Can you work these out from the model? Positions are in its coordinate system, mm. A direction names the side the tool comes from. Give positions to 0.01 mm unless a question says otherwise; leave off trailing zeros. Loops run counter-clockwise (first coordinate to the right, second up) from the corner with the lowest first, then second, coordinate; pieces in that order, holes last. Notation, with made-up numbers: (53.25, -9.75) -> (57.25, -9.75) arc R13 ccw to (57.25, 7.25) -> close; hole circle Ø9 at (-12, 11). An arc over 180 degrees is marked (long way). One line per question, with ' | ' between items.
from build123d import *

# Parameters (mm, degrees)
BOSS_EXTRUDE1_DEPTH     = 8
FILL_PATTERN1_OUTLINE_R = 2.75
FILL_PATTERN1_DEPTH     = 8


# Read off the part's stored shape, not the designer's step: Fill Pattern1
with BuildPart() as part:
    # Sketch1 → Boss-Extrude1 (new body)
    with BuildSketch(Plane.XY):
        with BuildLine():
            Line((-145, -2.75), (-145, -72.5))
            Line((-145, -72.5), (-2.75, -72.5))
            Line((-2.75, -72.5), (-2.75, -47.5))
            ThreePointArc((-2.75, -47.5), (0, -44.75), (2.75, -47.5))
            Line((2.75, -47.5), (2.75, -72.5))
            Line((2.75, -72.5), (145, -72.5))
            Line((145, -72.5), (145, -2.75))
            Line((145, -2.75), (120, -2.75))
            ThreePointArc((120, -2.75), (117.25, 0), (120, 2.75))
            Line((120, 2.75), (145, 2.75))
            Line((145, 2.75), (145, 72.5))
            Line((145, 72.5), (2.75, 72.5))
            Line((2.75, 72.5), (2.75, 47.5))
            ThreePointArc((2.75, 47.5), (0, 44.75), (-2.75, 47.5))
            Line((-2.75, 47.5), (-2.75, 72.5))
            Line((-2.75, 72.5), (-145, 72.5))
            Line((-145, 72.5), (-145, 2.75))
            Line((-145, 2.75), (-120, 2.75))
            ThreePointArc((-120, 2.75), (-117.25, 0), (-120, -2.75))
            Line((-120, -2.75), (-145, -2.75))
        make_face()
        with BuildLine():
            ThreePointArc((-43.840620434, 41.012193309), (-43.840620434, 43.840620434), (-41.012193309, 43.840620434))
            Line((-41.012193309, 43.840620434), (0, 2.828427125))
            Line((0, 2.828427125), (41.012193309, 43.840620434))
            ThreePointArc((41.012193309, 43.840620434), (43.840620434, 43.840620434), (43.840620434, 41.012193309))
            Line((43.840620434, 41.012193309), (2.828427125, 0))
            Line((2.828427125, 0), (43.840620434, -41.012193309))
            ThreePointArc((43.840620434, -41.012193309), (43.840620434, -43.840620434), (41.012193309, -43.840620434))
            Line((41.012193309, -43.840620434), (0, -2.828427125))
            Line((0, -2.828427125), (-41.012193309, -43.840620434))
            ThreePointArc((-41.012193309, -43.840620434), (-43.840620434, -43.840620434), (-43.840620434, -41.012193309))
            Line((-43.840620434, -41.012193309), (-2.828427125, 0))
            Line((-2.828427125, 0), (-43.840620434, 41.012193309))
        make_face(mode=Mode.SUBTRACT)
        Polygon((-50, -13.856406461), (-58, 0), (-50, 13.856406461), (-34, 13.856406461), (-26, 0), (-34, -13.856406461), align=None, mode=Mode.SUBTRACT)
        Polygon((50, 13.856406461), (58, 0), (50, -13.856406461), (34, -13.856406461), (26, 0), (34, 13.856406461), align=None, mode=Mode.SUBTRACT)
    extrude(amount=BOSS_EXTRUDE1_DEPTH)

    # Fill Pattern1 outline → Fill Pattern1 (cut)
    with BuildSketch(Plane.XY):
        with Locations((50, 50)):
            Circle(FILL_PATTERN1_OUTLINE_R)
        with Locations((-50, 25)):
            Circle(FILL_PATTERN1_OUTLINE_R)
        with Locations((-50, -25)):
            Circle(FILL_PATTERN1_OUTLINE_R)
        with Locations((-50, -50)):
            Circle(FILL_PATTERN1_OUTLINE_R)
        with Locations((125, -50)):
            Circle(FILL_PATTERN1_OUTLINE_R)
        with Locations((-25, -50)):
            Circle(FILL_PATTERN1_OUTLINE_R)
        with Locations((0, 25)):
            Circle(FILL_PATTERN1_OUTLINE_R)
        with Locations((125, -25)):
            Circle(FILL_PATTERN1_OUTLINE_R)
        with Locations((100, -50)):
            Circle(FILL_PATTERN1_OUTLINE_R)
        with Locations((25, 50)):
            Circle(FILL_PATTERN1_OUTLINE_R)
        with Locations((-75, 0)):
            Circle(FILL_PATTERN1_OUTLINE_R)
        with Locations((-75, 25)):
            Circle(FILL_PATTERN1_OUTLINE_R)
        with Locations((-75, 50)):
            Circle(FILL_PATTERN1_OUTLINE_R)
        with Locations((-75, -25)):
            Circle(FILL_PATTERN1_OUTLINE_R)
        with Locations((-75, -50)):
            Circle(FILL_PATTERN1_OUTLINE_R)
        with Locations((-25, 50)):
            Circle(FILL_PATTERN1_OUTLINE_R)
        with Locations((-50, 50)):
            Circle(FILL_PATTERN1_OUTLINE_R)
        with Locations((100, 25)):
            Circle(FILL_PATTERN1_OUTLINE_R)
        with Locations((75, 0)):
            Circle(FILL_PATTERN1_OUTLINE_R)
        with Locations((50, -25)):
            Circle(FILL_PATTERN1_OUTLINE_R)
        with Locations((0, -25)):
            Circle(FILL_PATTERN1_OUTLINE_R)
        with Locations((50, 25)):
            Circle(FILL_PATTERN1_OUTLINE_R)
        with Locations((75, 50)):
            Circle(FILL_PATTERN1_OUTLINE_R)
        with Locations((75, 25)):
            Circle(FILL_PATTERN1_OUTLINE_R)
        with Locations((100, 50)):
            Circle(FILL_PATTERN1_OUTLINE_R)
        with Locations((125, 25)):
            Circle(FILL_PATTERN1_OUTLINE_R)
        with Locations((25, -50)):
            Circle(FILL_PATTERN1_OUTLINE_R)
        with Locations((75, -50)):
            Circle(FILL_PATTERN1_OUTLINE_R)
        with Locations((100, -25)):
            Circle(FILL_PATTERN1_OUTLINE_R)
        with Locations((125, 50)):
            Circle(FILL_PATTERN1_OUTLINE_R)
        with Locations((50, -50)):
            Circle(FILL_PATTERN1_OUTLINE_R)
        with Locations((75, -25)):
            Circle(FILL_PATTERN1_OUTLINE_R)
        with Locations((100, 0)):
            Circle(FILL_PATTERN1_OUTLINE_R)
        with Locations((-125, 50)):
            Circle(FILL_PATTERN1_OUTLINE_R)
        with Locations((-100, -50)):
            Circle(FILL_PATTERN1_OUTLINE_R)
        with Locations((-100, -25)):
            Circle(FILL_PATTERN1_OUTLINE_R)
        with Locations((-100, 0)):
            Circle(FILL_PATTERN1_OUTLINE_R)
        with Locations((-100, 25)):
            Circle(FILL_PATTERN1_OUTLINE_R)
        with Locations((-125, 25)):
            Circle(FILL_PATTERN1_OUTLINE_R)
        with Locations((-125, -25)):
            Circle(FILL_PATTERN1_OUTLINE_R)
        with Locations((-125, -50)):
            Circle(FILL_PATTERN1_OUTLINE_R)
        with Locations((-100, 50)):
            Circle(FILL_PATTERN1_OUTLINE_R)
    extrude(amount=FILL_PATTERN1_DEPTH, mode=Mode.SUBTRACT)


solid = part.part
Q1. For pin 1 Ø3.5 at (x, y) = (50, -50) entering from +Z, with a flat end and sliding along its axis, tell me the tip position at first contact or that it passes through.
Entries:
pin 1: through
Q2. If we section it at C-C (z = 4.5): State how many separate pieces and enclosed holes the cut face has, plus the area to 3 significant figures.
Entries:
separate pieces: 1 | enclosed holes: 45 | area: 38,200 mm²
Q3. On a 3-axis mill with a long thin cutter (end or side, diameter ignored), from which of +Z, -Z, +X, -X, +Y, -Y can I reach the whole of each face in a straight line? I mean faces 4 (the face through (2.75, -60, 4)), 5 (the face through (-53.94, -7.03, 3.94)), 6 (the face through (2.75, 60, 4)). Say none if no direction works.
Entries:
face 4: +Z, -Z, -Y | face 5: +Z, -Z | face 6: +Z, -Z, +Y
Q4. If we section it at A-A (y = -59.5): Write out the boundary of the cut face in (x, z).
Entries:
outline: (-145, 0) -> (-2.75, 0) -> (-2.75, 8) -> (-145, 8) -> close; (2.75, 0) -> (145, 0) -> (145, 8) -> (2.75, 8) -> close
Q5. If we mould it in two halves opening along Y, with no side actions, what happens to faces 1 (the face through (42, -13.856, 4)), 2 (the face through (-0.06, -44.75, 3.94)), 3 (the face through (-145, -37, 4))? For each: pulls with the +Y half, pulls with the -Y half, needs draft (parallel to the pull), parting line crosses it, or undercut.
Entries:
face 1: undercut | face 2: pulls with the -Y half | face 3: needs draft
Q6. If I drill on probe 1 along Y at (x, z) = (50, 3.25); probe 2 along Y at (x, z) = (125, 7.5); probe 3 along X at (y, z) = (63, 1.5), over which ranges is the centre line in solid material (lowest first)? Write a range as from..to.
Entries:
probe 1: -72.5..-52.75, -47.25..-27.75, -22.25..-13.86, 13.86..22.25, 27.75..47.25, 52.75..72.5 | probe 2: -72.5..-52.75, -47.25..-27.75, -22.25..-2.75, 2.75..22.25, 27.75..47.25, 52.75..72.5 | probe 3: -145..-2.75, 2.75..145
Q7. If we section it at B-B (x = 125): Write out the boundary of the cut face in (y, z), plus the area to 3 significant figures.
Entries:
outline: (-72.5, 0) -> (-52.75, 0) -> (-52.75, 8) -> (-72.5, 8) -> close; (-47.25, 0) -> (-27.75, 0) -> (-27.75, 8) -> (-47.25, 8) -> close; (-22.25, 0) -> (-2.75, 0) -> (-2.75, 8) -> (-22.25, 8) -> close; (2.75, 0) -> (22.25, 0) -> (22.25, 8) -> (2.75, 8) -> close; (27.75, 0) -> (47.25, 0) -> (47.25, 8) -> (27.75, 8) -> close; (52.75, 0) -> (72.5, 0) -> (72.5, 8) -> (52.75, 8) -> close | area: 940 mm²
